```python
from build123d import *

# Parameters (mm, degrees)
PAD_DEPTH       = 80
POCKET_START    = -7
SKETCH001_R     = 9.5
POCKET_DEPTH    = 66
SKETCH007_R     = 3.1
POCKET005_DEPTH = 5
POCKET006_START = -10
POCKET006_DEPTH = 60
SKETCH009_R     = 1.75
POCKET007_DEPTH = 13.001
SKETCH010_W     = 22
SKETCH010_H     = 8
POCKET008_DEPTH = 11
SKETCH011_R     = 1.5
POCKET009_DEPTH = 5
SKETCH012_R     = 2.75
POCKET010_DEPTH = 3
SKETCH013_R     = 2.5
POCKET011_DEPTH = 80.001
POCKET012_START = -2
SKETCH014_W     = 23
SKETCH014_H     = 7
POCKET012_DEPTH = 76
POCKET013_DEPTH = 0.3
POCKET014_DEPTH = 0.3


with BuildPart() as part:
    # Sketch → Pad (new body)
    with BuildSketch(Plane.YZ):
        with BuildLine():
            Line((0, 0), (60, 0))
            Line((60, 0), (60, -4))
            ThreePointArc((51, -13), (57.363961, -10.363961), (60, -4))
            Line((51, -13), (9, -13))
            ThreePointArc((0, -4), (2.636039, -10.363961), (9, -13))
            Line((0, -4), (0, 0))
        make_face()
    extrude(amount=PAD_DEPTH)

    # Sketch001 (on Face8 of Pad) → Pocket (cut)
    with BuildSketch(Plane.YZ.offset(80).offset(POCKET_START)):
        with Locations((12.5, 0)):
            Circle(SKETCH001_R)
    extrude(amount=-POCKET_DEPTH, mode=Mode.SUBTRACT)

    # Sketch007 → Pocket005 (cut)
    with BuildSketch(Plane.ZX.offset(60)):
        with Locations((0, 51)):
            Circle(SKETCH007_R)
        with Locations((0, 36)):
            Circle(SKETCH007_R)
        with Locations((0, 21)):
            Circle(SKETCH007_R)
    extrude(amount=-POCKET005_DEPTH, mode=Mode.SUBTRACT)

    # Sketch008 (on Face5 of Pocket005) → Pocket006 (cut)
    with BuildSketch(Plane.YZ.offset(80).offset(POCKET006_START)):
        with BuildLine():
            Line((57, 0), (25, 0))
            Line((25, 0), (25, -11))
            Line((25, -11), (51, -11))
            ThreePointArc((51, -11), (55.242641, -9.242641), (57, -5))
            Line((57, -5), (57, 0))
        make_face()
    extrude(amount=-POCKET006_DEPTH, mode=Mode.SUBTRACT)

    # Sketch009 (on Face3 of Pocket006) → Pocket007 (cut, through all)
    with BuildSketch(Plane(origin=(0, 0, 0), x_dir=(0, -1, 0), z_dir=(0, 0, 1))):
        with Locations((-51, 74.1)):
            Circle(SKETCH009_R)
        with Locations((-10, 75.5)):
            Circle(SKETCH009_R)
        with Locations((-51, 6.1)):
            Circle(SKETCH009_R)
        with Locations((-10, 4.5)):
            Circle(SKETCH009_R)
    extrude(amount=-POCKET007_DEPTH, mode=Mode.SUBTRACT)

    # Sketch010 (on Face3 of Pocket007) → Pocket008 (cut)
    with BuildSketch(Plane(origin=(0, 0, 0), x_dir=(0, -1, 0), z_dir=(0, 0, 1))):
        with Locations((-36, 74)):
            Rectangle(SKETCH010_W, SKETCH010_H)
        with Locations((-36, 6)):
            Rectangle(SKETCH010_W, SKETCH010_H)
    extrude(amount=-POCKET008_DEPTH, mode=Mode.SUBTRACT)

    # Sketch011 (on Face6 of Pocket008) → Pocket009 (cut)
    with BuildSketch(Plane.YX.offset(13)):
        with Locations((51, 60.1)):
            Circle(SKETCH011_R)
        with Locations((45, 60.1)):
            Circle(SKETCH011_R)
    extrude(amount=-POCKET009_DEPTH, mode=Mode.SUBTRACT)

    # Sketch012 (on Face6 of Pocket009) → Pocket010 (cut)
    with BuildSketch(Plane.YX.offset(13)):
        with Locations((51, 6.1)):
            Circle(SKETCH012_R)
        with Locations((10, 4.5)):
            Circle(SKETCH012_R)
        with Locations((10, 75.5)):
            Circle(SKETCH012_R)
        with Locations((51, 74.1)):
            Circle(SKETCH012_R)
    extrude(amount=-POCKET010_DEPTH, mode=Mode.SUBTRACT)

    # Sketch013 (on Face4 of Pocket010) → Pocket011 (cut, through all)
    with BuildSketch(Plane(origin=(0, 0, 0), x_dir=(0, 1, 0), z_dir=(-1, 0, 0))):
        with Locations((37, 4)):
            Circle(SKETCH013_R)
    extrude(amount=-POCKET011_DEPTH, mode=Mode.SUBTRACT)

    # Sketch014 (on Face4 of Pocket011) → Pocket012 (cut)
    with BuildSketch(Plane(origin=(0, 0, 0), x_dir=(0, 1, 0), z_dir=(-1, 0, 0)).offset(POCKET012_START)):
        with Locations((14.5, 0)):
            Rectangle(SKETCH014_W, SKETCH014_H)
    extrude(amount=-POCKET012_DEPTH, mode=Mode.SUBTRACT)

    # Sketch015 (on Face6 of Pocket012) → Pocket013 (cut)
    with BuildSketch(Plane.YX.offset(13)):
        Polygon((43.5, 57.698076), (45, 55.1), (46.5, 57.698076), align=None)
    extrude(amount=-POCKET013_DEPTH, mode=Mode.SUBTRACT)

    # Sketch016 (on Face6 of Pocket013) → Pocket014 (cut)
    with BuildSketch(Plane.YX.offset(13)):
        Polygon((47.5, 62.501924), (50.5, 62.501924), (49, 65.1), align=None)
    extrude(amount=-POCKET014_DEPTH, mode=Mode.SUBTRACT)


solid = part.part
```
For this review, take the finished solid that the model builds, in its own axes (mm). A direction names the side the tool comes from. Round coordinates to 2 decimals unless told otherwise and drop trailing zeros. Write each loop counter-clockwise with the first axis right and the second up, starting at its lowest first coordinate (ties: lowest second). Pieces come first, ordered by that corner, then holes. Notation, with made-up numbers: (25, -4) -> (34, -4) arc R9 cw to (34, 7) -> close; hole circle Ø9 at (20.25, 77). An arc over 180 degrees is marked (long way). Use one line per item in the form item = value.
Q1. To check wall thickness, follow probe 1 along X at (y, z) = (51, -2.75); probe 2 along X at (y, z) = (10, -7.5); probe 3 along Y at (x, z) = (58, -7). State the ranges of each line that lie inside material, in increasing order. Write a range as from..to.
Resolved:
probe_1 = 0..4.35, 7.85..10, 70..72.35, 75.85..80
probe_2 = 0..2.75, 6.25..7, 73..73.75, 77.25..80
probe_3 = 0.51..6.08, 18.92..25, 56.66..59.49
Q2. The part is to be moulded in two halves that separate along X. For faces 4 (the flat face through (39, 0, -2)), 5 (the flat face through (74, 47, -5)), 6 (the cylindrical face through (6.221, 48.253, -11.521)), 7 (the flat face through (0, 30, -6)), say which applies: released by +X, released by -X, zero draft, split by the parting line, or undercut.
Resolved:
face_4 = zero draft
face_5 = undercut
face_6 = undercut
face_7 = released by -X
Q3. Consider section B-B (y = 37). State the section outline as (x, z) points.
Resolved:
outline = (0, -13) -> (80, -13) -> (80, -6.5) -> (78, -6.5) -> (78, -11) -> (2, -11) -> (2, -6.5) -> (0, -6.5) -> close; (0, -1.5) -> (2, -1.5) -> (2, 0) -> (0, 0) -> close; (78, -1.5) -> (80, -1.5) -> (80, 0) -> (78, 0) -> close
Q4. Clearance check with flat-ended pins moving along their axes: pin 1 Ø3 at (x, y) = (19, 8.5) entering from -Z; pin 2 Ø5 at (x, z) = (17.5, -10) entering from -Y; pin 3 Ø5 at (x, y) = (4.5, 10) entering from -Z; pin 4 Ø6 at (x, z) = (48, -9) entering from +Y. State where each tip first meets the part, or that it passes through.
Resolved:
pin_1 = -13
pin_2 = 0.71
pin_3 = -10
pin_4 = 59.77
Q5. Consider section A-A (x = 21). State the section outline as (y, z) points, then the cut area to 3 significant figures.
Resolved:
outline = (0, -4) arc R9 ccw to (9, -13) -> (51, -13) arc R9 ccw to (60, -4) -> (60, -3.1) -> (57, -3.1) -> (57, -5) arc R6 cw to (51, -11) -> (25, -11) -> (25, -3.5) -> (21.33, -3.5) arc R9.5 cw to (3.67, -3.5) -> (3, -3.5) -> (3, 0) -> (0, 0) -> close
area = 238 mm²
Q6. Machinability: for faces 1 (the cylindrical face through (21.1, 58.5, -3.1)), 2 (the flat face through (40, 57, -3)), 3 (the flat face through (57, 45, -12.7)), which of the approach directions +Z, -Z, +X, -X, +Y, -Y give a long, thin tool a straight path to every point of the face, cutting with its end or side? Answer none if there is none.
Resolved:
face_1 = +Z, +Y
face_2 = +Z
face_3 = -Z
Q7. Consider section C-C (x = 60.1). State the section outline as (y, z) points.
Resolved:
outline = (0, -4) arc R9 ccw to (9, -13) -> (43.5, -13) -> (43.5, -11) -> (25, -11) -> (25, -3.5) -> (21.33, -3.5) arc R9.5 cw to (3.67, -3.5) -> (3, -3.5) -> (3, 0) -> (0, 0) -> close; (46.5, -13) -> (49.5, -13) -> (49.5, -11) -> (46.5, -11) -> close; (52.5, -12.87) arc R9 ccw to (60, -4) -> (60, 0) -> (57, 0) -> (57, -5) arc R6 cw to (52.5, -10.81) -> close
Q8. Consider section D-D (z = -7.75). State the section outline as (x, y) points, then the cut area to 3 significant figures.
Resolved:
outline = (0, 0.82) -> (80, 0.82) -> (80, 59.18) -> (0, 59.18) -> close; hole (2, 25) -> (78, 25) -> (78, 47) -> (70, 47) -> (70, 56.33) -> (10, 56.33) -> (10, 47) -> (2, 47) -> close; hole circle Ø3.5 at (4.5, 10); hole circle Ø3.5 at (6.1, 51); hole (7, 7.01) -> (73, 7.01) -> (73, 17.99) -> (7, 17.99) -> close; hole circle Ø3.5 at (74.1, 51); hole circle Ø3.5 at (75.5, 10)
area = 1,670 mm²
